Geometry check sheet. Reference: drawing and pictorial views, mm from the part's lowest x, y, z. A direction names the side the tool comes from. Round coordinates to 2 decimals unless told otherwise and drop trailing zeros. Write each loop counter-clockwise with the first axis right and the second up, starting at its lowest first coordinate (ties: lowest second). Pieces come first, ordered by that corner, then holes. Notation, with made-up numbers: (10.5, -31.5) - (14.5, -31.5) arc R13 ccw to (14.5, -9.5) - close; hole circle Ø8 at (5.5, 85.5). An arc over 180 degrees is marked (long way). Return JSON: item names as keys, results as strings.
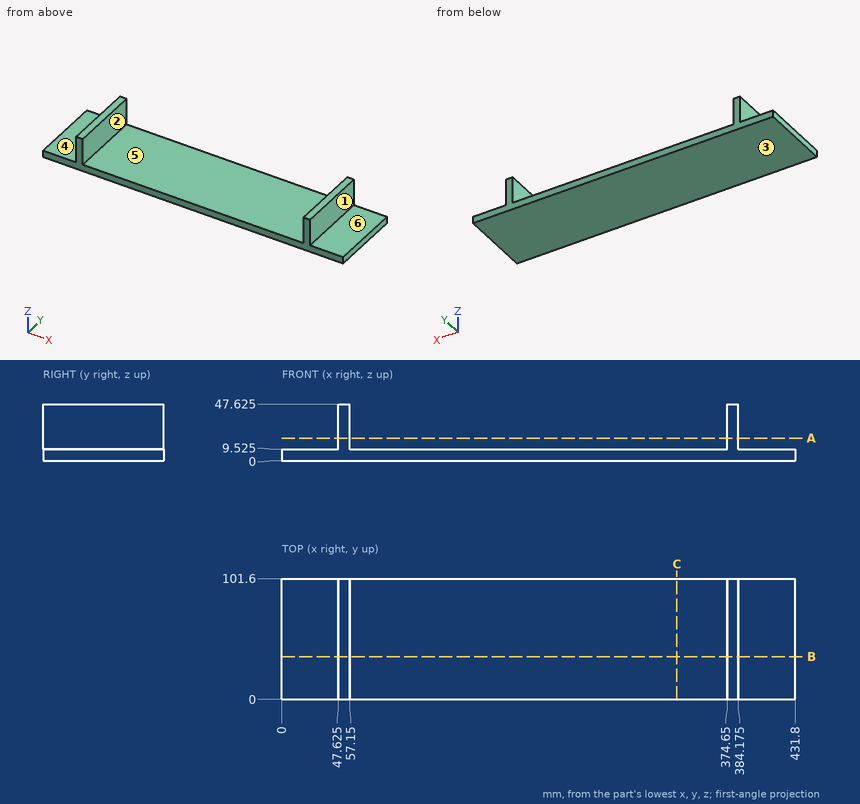
(1) Access from +Z, -Z, +X, -X, +Y, -Y to the whole of each face (thin tool, end or side, straight path). Record for the marked faces 4, 5 and 6.
Response values:
{"face 4": "+Z, -X, +Y, -Y", "face 5": "+Z, +Y, -Y", "face 6": "+Z, +X, +Y, -Y"}
(2) Material ranges on line 1 along X through (y, z) = (85, 41) (3 decimals); line 2 along Z through (x, y) = (82, 92) (3 decimals), recorded low to high. Write a range as [from, to].
Response values:
{"line 1": "x = [47.625, 57.15], [374.65, 384.175]", "line 2": "z = [0, 9.525]"}
(3) Section check B-B, the plane y = 36. Enter the section's corners in (x, z) (3 decimals).
Response values:
{"outline": "(0, 0) - (431.8, 0) - (431.8, 9.525) - (384.175, 9.525) - (384.175, 47.625) - (374.65, 47.625) - (374.65, 9.525) - (57.15, 9.525) - (57.15, 47.625) - (47.625, 47.625) - (47.625, 9.525) - (0, 9.525) - close"}
(4) Section check A-A, the plane z = 19. Enter the section's corners in (x, y) (3 decimals), plus the area to 3 significant figures.
Response values:
{"outline": "(47.625, 0) - (57.15, 0) - (57.15, 101.6) - (47.625, 101.6) - close; (374.65, 0) - (384.175, 0) - (384.175, 101.6) - (374.65, 101.6) - close", "area": "1,940 mm^2"}
(5) Section check C-C, the plane x = 332.5. Enter the section's corners in (y, z) (3 decimals), plus the area to 3 significant figures.
Response values:
{"outline": "(0, 0) - (101.6, 0) - (101.6, 9.525) - (0, 9.525) - close", "area": "968 mm^2"}
(6) Gauge pin test, flat ends, axial feed: pin 1 (3 mm diameter, centred on x = 44, y = 76.5, fed in from +Z) (3 decimals); pin 2 (11.5 mm diameter, centred on y = 58, z = 31, fed in from +X) (3 decimals); pin 3 (10 mm diameter, centred on y = 48, z = 16, fed in from -X) (3 decimals). Record the tip position at first contact, or that the pin passes through.
Response values:
{"pin 1": "stops at z = 9.525", "pin 2": "stops at x = 384.175", "pin 3": "stops at x = 47.625"}
(7) Release check for a two-part mould opening along X. For the marked faces 1, 2 and 3 record: pulls with the +X half, pulls with the -X half, needs draft (parallel to the pull), parting line crosses it, or undercut.
Response values:
{"face 1": "pulls with the +X half", "face 2": "undercut", "face 3": "needs draft"}
